from build123d import *

# Parameters (mm, degrees)
SKETCH_1_R          = 5.6
SKETCH_1_R_2        = 4.6
EXTRUDE_1_DEPTH     = 31.22
SKETCH_2_W          = 4.086350381
SKETCH_2_H          = 1
CUT_EXTRUDE_1_DEPTH = 33.208824878
FILLET_1_R          = 0.5


with BuildPart() as part:
    # 스케치1 → 보스-돌출1 (new body)
    with BuildSketch(Plane.XY):
        Circle(SKETCH_1_R)
        Circle(SKETCH_1_R_2, mode=Mode.SUBTRACT)
    extrude(amount=EXTRUDE_1_DEPTH)

    # 스케치2 → 컷-돌출1 (cut, through all)
    with BuildSketch(Plane.XY):
        with Locations((5.169276946, 0)):
            Rectangle(SKETCH_2_W, SKETCH_2_H)
    extrude(amount=CUT_EXTRUDE_1_DEPTH, mode=Mode.SUBTRACT)

    # 필렛1
    fillet_1_edges = [part.edges().sort_by_distance(p)[0] for p in [
        (4.572745346, -0.5, 15.61),
        (5.577633907, -0.5, 15.61),
        (5.577633907, 0.5, 15.61),
        (4.572745346, 0.5, 15.61),
    ]]
    fillet(fillet_1_edges, radius=FILLET_1_R - 0.0001)  # a hair under: the kernel refuses the full size


solid = part.part
Read the model definition and answer for the solid it produces. Units are mm, in the model's axes. Give positions to 0.01 mm unless a question says otherwise; leave off trailing zeros. Write each loop counter-clockwise with the first axis right and the second up, starting at its lowest first coordinate (ties: lowest second). Pieces come first, ordered by that corner, then holes. Notation, with made-up numbers: (84, 68.5) - (101, 68.5) arc R30 ccw to (101, 98.5) - close; hole circle Ø9 at (57, 66.25). An arc over 180 degrees is marked (long way). Answer in a Markdown table with one row per item. Add a question column.
Item 1: Determine the mould class of faces 1 (the face through (-4.596, 0.19, 15.391)), 2 (the face through (-5, 1, 0)), 3 (the face through (-5.595, 0.231, 15.391)) for opening direction X: pulls with the +X half, pulls with the -X half, needs draft (parallel to the pull), parting line crosses it, or undercut.
Item 2: Flat-ended cylindrical pins translate along their axes: P1, Ø1.5, axis at x = 1, z = 24.5, coming from the +Y side; P2, Ø3, axis at x = 2, z = 3.5, coming from the -Y side. Find the tip coordinate at first contact, or state that the pin passes through.
Item 3: Section B-B, the plane y = -1.5 is taken. Write down the section's boundary in (x, z), and give its area (3 significant figures).
Item 4: Section A-A, the plane x = 0 is taken. Write down the section's boundary in (y, z).
Item 5: Find the intervals of material crossed by L1, parallel to Y at x = 0, z = 12; L2, parallel to X at y = 0, z = 17; L3, parallel to X at y = 1, z = 25, in increasing order.
Recorded:
| question | item | result |
|---|---|---|
| 1 | face 1 | undercut |
| 1 | face 2 | needs draft |
| 1 | face 3 | parting line crosses it |
| 2 | P1 | stops at y = 5.59 |
| 2 | P2 | stops at y = -5.58 |
| 3 | outline | (-5.4, 0) - (-4.35, 0) - (-4.35, 31.22) - (-5.4, 31.22) - close; (4.35, 0) - (5.4, 0) - (5.4, 31.22) - (4.35, 31.22) - close |
| 3 | area | 65.4 mm2 |
| 4 | outline | (-5.6, 0) - (-4.6, 0) - (-4.6, 31.22) - (-5.6, 31.22) - close; (4.6, 0) - (5.6, 0) - (5.6, 31.22) - (4.6, 31.22) - close |
| 5 | L1 | y = -5.6 to -4.6, 4.6 to 5.6 |
| 5 | L2 | x = -5.6 to -4.6 |
| 5 | L3 | x = -5.51 to -4.49, 4.49 to 5.5 |
